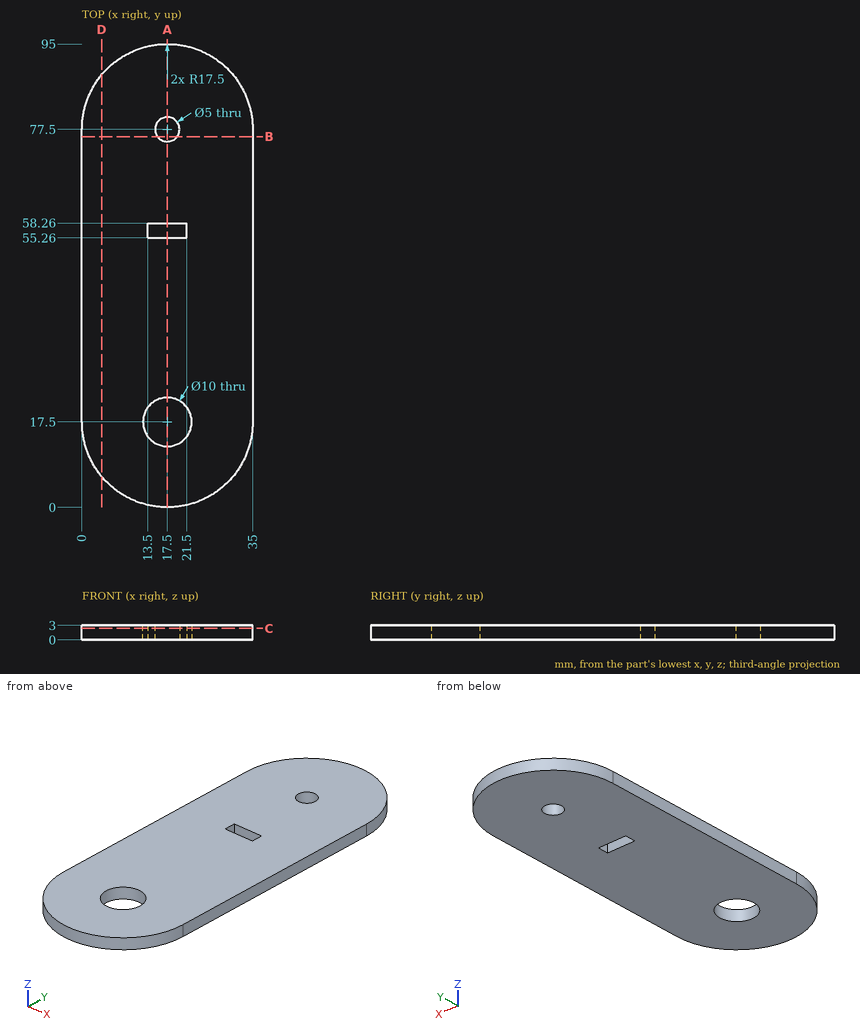
The figure shows three views and two pictorial views of one solid part (mm, origin at its lowest corner). Answer the questions. Coordinates: 2 decimals unless noted, no trailing zeros. Write each loop counter-clockwise with the first axis right and the second up, starting at its lowest first coordinate (ties: lowest second). Pieces come first, ordered by that corner, then holes.
1. Flat-ended cylindrical pins translate along their axes: pin 1 (1.5 mm diameter, centred on x = 14, z = 2.5, fed in from +Y); pin 2 (1 mm diameter, centred on x = 22.5, z = 0.5, fed in from -Y). Find the tip coordinate at first contact, or state that the pin passes through.
Results list:
pin 1: stops at y = 94.78
pin 2: stops at y = 0.59
2. The part is cut by section A-A, the plane x = 17.5. Write down the section's boundary in (y, z).
Results list:
outline: (0, 0) - (12.5, 0) - (12.5, 3) - (0, 3) - close; (22.5, 0) - (55.26, 0) - (55.26, 3) - (22.5, 3) - close; (58.26, 0) - (75, 0) - (75, 3) - (58.26, 3) - close; (80, 0) - (95, 0) - (95, 3) - (80, 3) - close
3. The part is cut by section D-D, the plane x = 4. Write down the section's boundary in (y, z), and give its area (3 significant figures).
Results list:
outline: (6.36, 0) - (88.64, 0) - (88.64, 3) - (6.36, 3) - close
area: 247 mm2
4. The part is cut by section B-B, the plane y = 76. Write down the section's boundary in (x, z).
Results list:
outline: (0, 0) - (15.5, 0) - (15.5, 3) - (0, 3) - close; (19.5, 0) - (35, 0) - (35, 3) - (19.5, 3) - close
5. The part is cut by section C-C, the plane z = 2.35. Write down the section's boundary in (x, y).
Results list:
outline: (0, 17.5) arc R17.5 ccw to (35, 17.5) - (35, 77.5) arc R17.5 ccw to (0, 77.5) - close; hole circle Ø10 at (17.5, 17.5); hole (13.5, 55.26) - (21.5, 55.26) - (21.5, 58.26) - (13.5, 58.26) - close; hole circle Ø5 at (17.5, 77.5)
6. Consider line 1 along Y through (x, z) = (17.5, 2.15); line 2 along X through (y, z) = (77.5, 2.4); line 3 along Y through (x, z) = (14, 1.25). Determine where each line is inside the solid, lowest interval first.
Results list:
line 1: y = 0 to 12.5, 22.5 to 55.26, 58.26 to 75, 80 to 95
line 2: x = 0 to 15, 20 to 35
line 3: y = 0.35 to 13.93, 21.07 to 55.26, 58.26 to 94.65
